Could you check a few things on this model? Use its own coordinates, in mm. Face numbers are marked on the shaded views. Give positions to 0.01 mm unless a question says otherwise; leave off trailing zeros. Loops run counter-clockwise (first coordinate to the right, second up) from the corner with the lowest first, then second, coordinate; pieces in that order, holes last. Notation, with made-up numbers: M -2,35 L 5,35 A19 cw 5,46 Z; hole C -37,-28.5 d10. An arc over 180 degrees is marked long. Return JSON: item names as keys, results as strings. Group by question number.
1. If we mould it in two halves opening along Z, with no side actions, what happens to the marked faces 1, 2 and 3? For each: +Z half, -Z half, draft (parallel to the pull), parting line (faces both ways), or undercut.
2. If we section it at A-A (x = 0): Write out the boundary of the cut face in (y, z).
3. If we section it at D-D (z = 0): Write out the boundary of the cut face in (x, y), plus the area to 4 significant figures.
4. If we section it at B-B (z = -22): Write out the boundary of the cut face in (x, y), plus the area to 3 significant figures.
5. Please list where these lines run through material, in increasing order: line 1 (Z direction, x = 0, y = -4); line 2 (Z direction, x = -3, y = -3); line 3 (Z direction, x = -6.25, y = -1.25).
6. For pin 1 (7 mm diameter, centred on x = 0, z = 0, fed in from +Y), with a flat end and sliding along its axis, tell me the tip position at first contact or that it passes through.
7. If we section it at C-C (y = -5.75): Write out the boundary of the cut face in (x, z).
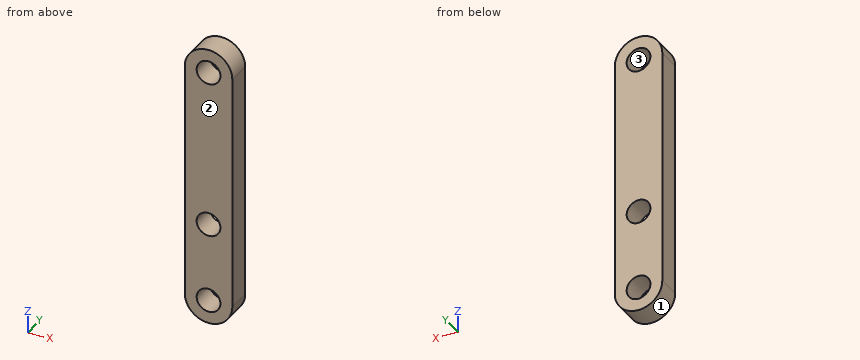
```python
from build123d import *

# Parameters (mm, degrees)
F0_R     = 3.75
F1_DEPTH = 7.62


with BuildPart() as f1:
    # F0 (on Front) → F1 (new body)
    with BuildSketch(Plane.XZ):
        with BuildLine():
            ThreePointArc((-7.5, -25), (0, -32.5), (7.5, -25))
            ThreePointArc((7.5, -25), (0, -17.5), (-7.5, -25))
        make_face()
        with Locations((0, -25)):
            Circle(F0_R, mode=Mode.SUBTRACT)
        with BuildLine():
            ThreePointArc((-7.5, -25), (0, -17.5), (7.5, -25))
            Line((7.5, -25), (7.5, 50))
            ThreePointArc((7.5, 50), (0, 42.5), (-7.5, 50))
            Line((-7.5, 50), (-7.5, -25))
        make_face()
        Circle(F0_R, mode=Mode.SUBTRACT)
        with BuildLine():
            ThreePointArc((-7.5, 50), (0, 42.5), (7.5, 50))
            ThreePointArc((7.5, 50), (0, 57.5), (-7.5, 50))
        make_face()
        with Locations((0, 50)):
            Circle(F0_R, mode=Mode.SUBTRACT)
    extrude(amount=F1_DEPTH)


solid = f1.part
```
Answer:
{
 "1": {"face 1": "-Z half", "face 2": "draft", "face 3": "undercut"},
 "2": {"outline": "M -7.62,-32.5 L 0,-32.5 L 0,-28.75 L -7.62,-28.75 Z; M -7.62,-21.25 L 0,-21.25 L 0,-3.75 L -7.62,-3.75 Z; M -7.62,3.75 L 0,3.75 L 0,46.25 L -7.62,46.25 Z; M -7.62,53.75 L 0,53.75 L 0,57.5 L -7.62,57.5 Z"},
 "3": {"outline": "M -7.5,-7.62 L -3.75,-7.62 L -3.75,0 L -7.5,0 Z; M 3.75,-7.62 L 7.5,-7.62 L 7.5,0 L 3.75,0 Z", "area": "57.15 mm²"},
 "4": {"outline": "M -7.5,-7.62 L -2.25,-7.62 L -2.25,0 L -7.5,0 Z; M 2.25,-7.62 L 7.5,-7.62 L 7.5,0 L 2.25,0 Z", "area": "80.0 mm²"},
 "5": {"line 1": "z = -32.5 to -28.75, -21.25 to -3.75, 3.75 to 46.25, 53.75 to 57.5", "line 2": "z = -31.87 to -27.25, -22.75 to -2.25, 2.25 to 47.75, 52.25 to 56.87", "line 3": "z = -29.15 to 54.15"},
 "6": {"pin 1": "passes through"},
 "7": {"outline": "M -7.5,-25 A7.5 ccw 7.5,-25 L 7.5,50 A7.5 ccw -7.5,50 Z; hole C 0,-25 d7.5; hole C 0,0 d7.5; hole C 0,50 d7.5"}
}
